Autodesk Inventor part; units mm, degrees
ref_plane "YZ Plane" through (0, 0, 0) normal (1, 0, 0) x (0, 1, 0)
ref_plane "XZ Plane" through (0, 0, 0) normal (0, 1, 0) x (-1, 0, 0)
ref_plane "XY Plane" through (0, 0, 0) normal (0, 0, 1) x (1, 0, 0)
sketch "Sketch1" plane through (0, 0, 0) normal (0, 0, 1) x (1, 0, 0)
  line L0 (-15.5765, 8.1) -> (15.5765, 8.1)
  line L1 (15.5765, 8.1) -> (15.5765, -8.1)
  line L2 (15.5765, -8.1) -> (-15.5765, -8.1)
  line L3 (-15.5765, -8.1) -> (-15.5765, 8.1)
  line L4 (0, 11.34) -> (0, -11.34) construction
  line L5 (-21.8071, 0) -> (21.8071, 0) construction
  point P0 (0, 0)
  dimension "d0" = 31.153
  dimension "d1" = 16.2
extrude "Extrusion1" add sketch "Sketch1" along normal blind 15
sketch "Sketch2" plane through (0, 0, 15) normal (0, 0, 1) x (1, 0, 0)
  line L0 (-15.5765, 8.1) -> (-15.5765, -8.1)
  circle A0 centre (-6.5765, 0) radius 5
  line L1 (-21.8071, 0) -> (21.8071, 0) construction
  point P0 (0, 0)
  dimension "d5" = 10
  dimension "d6" = 9
extrude "Extrusion2" cut sketch "Sketch2" against normal blind 10
properties part number "supporto_guide_10Z"
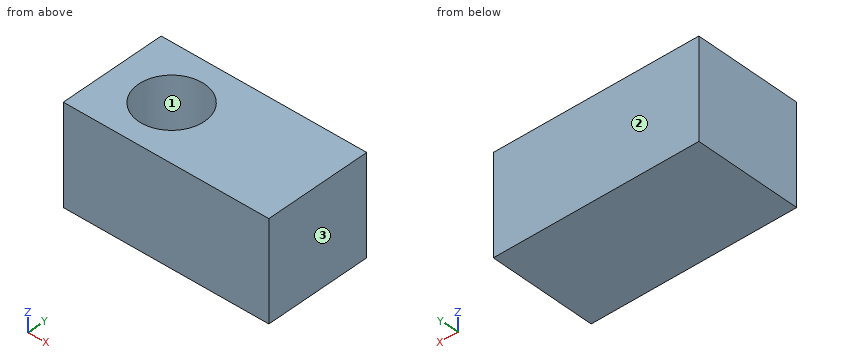
Source: CAD feature listing. Evaluate the final solid. Frame: model axes, mm. Face numbers are marked on the shaded views. Round coordinates to 2 decimals unless told otherwise and drop trailing zeros. Write each loop counter-clockwise with the first axis right and the second up, starting at its lowest first coordinate (ties: lowest second). Pieces come first, ordered by that corner, then holes. Notation, with made-up numbers: M 5,-14 L 23,-14 A10 cw 23,2 Z; hole C 86,32 d5. An arc over 180 degrees is marked long. Answer as a JSON object with one key per item and string values. Group by question number.
(1) Mould query, pull axis Y, two halves, no side actions, for the marked faces 1, 2 and 3. Classes: +Y half, -Y half, draft (parallel to the pull), parting line (faces both ways), or undercut.
(2) Section query C-C on x = -6. Output: boundary loops of the cut face in (y, z).
(3) First-contact query: pin 1 (8 mm diameter, centred on x = -7, y = 1.5, fed in from +Z). Flat tip, straight axial feed; report the tip coordinate or a pass-through.
(4) Ray query, line 1 (Y direction, x = -6.5, z = 6.75); line 2 (Z direction, x = -10, y = 1.5); line 3 (X direction, y = -2, z = 7.25). Return the intervals inside material, ascending. Write a range as [from, to].
(5) Section query B-B on z = 6.75. Output: boundary loops of the cut face in (x, y).
(6) Section query A-A on y = 0. Output: boundary loops of the cut face in (x, z), then the cut area to 3 significant figures.
Computed values:
{
 "1": {"face 1": "undercut", "face 2": "+Y half", "face 3": "draft"},
 "2": {"outline": "M -8.1,0 L 8.1,0 L 8.1,15 L 4.97,15 L 4.97,5 L -4.97,5 L -4.97,15 L -8.1,15 Z"},
 "3": {"pin 1": "z = 15"},
 "4": {"line 1": "[-8.1, -5], [5, 8.1]", "line 2": "[0, 5]", "line 3": "[-15.58, -11.16], [-1.99, 15.58]"},
 "5": {"outline": "M -15.58,-8.1 L 15.58,-8.1 L 15.58,8.1 L -15.58,8.1 Z; hole C -6.58,0 d10"},
 "6": {"outline": "M -15.58,0 L 15.58,0 L 15.58,15 L -1.58,15 L -1.58,5 L -11.58,5 L -11.58,15 L -15.58,15 Z", "area": "367 mm^2"}
}
